```python
from build123d import *

# Parameters (mm, degrees)
SKETCH1_W               = 229
SKETCH1_H               = 15
BOSS_EXTRUDE1_DEPTH     = 3.375
M3_CLEARANCE_HOLE1_D    = 3.4
CUT_EXTRUDE1_DEPTH      = 116.527661731
CUT_EXTRUDE1_DEPTH_BACK = 116.527661731
SKETCH10_W              = 15
SKETCH10_H              = 1.6875


with BuildPart() as part:
    # Sketch1 → Boss-Extrude1 (new body)
    with BuildSketch(Plane(origin=(0, 0, 0), x_dir=(1, 0, 0), z_dir=(0, 1, 0))):
        Rectangle(SKETCH1_W, SKETCH1_H)
    extrude(amount=BOSS_EXTRUDE1_DEPTH)

    # M3 Clearance Hole1 (through all)
    with Locations(Plane(origin=(0, 0, 0), x_dir=(-1, 0, 0), z_dir=(0, -1, 0))):
        with Locations((57, 0), (-57, 0)):
            Hole(M3_CLEARANCE_HOLE1_D / 2)

    # Sketch10 → Cut-Extrude1 (cut, two sides: drawn at the far end of the back side and taken through both)
    with BuildSketch(Plane.XY.offset(7.5).offset(-CUT_EXTRUDE1_DEPTH_BACK)):
        with Locations((0, 2.53125)):
            Rectangle(SKETCH10_W, SKETCH10_H)
    extrude(amount=CUT_EXTRUDE1_DEPTH + CUT_EXTRUDE1_DEPTH_BACK, mode=Mode.SUBTRACT)


solid = part.part
```
Geometry: final body of the model. Coordinates: model frame, mm. Coordinates: 2 decimals unless noted, no trailing zeros. Order: outer loops, then holes, each group sorted by start corner. A loop starts at its lowest first (then second) coordinate and runs counter-clockwise, first axis right, second up. Notation, with made-up numbers: (73.25, 28.5) - (125.25, 28.5) arc R31 cw to (125.25, 52.5) - close; hole circle Ø10 at (24.5, 13). An arc over 180 degrees is marked (long way). Write each question's results on one line, items separated by ' | '.
1) Section A-A, the plane z = 3.75. Return loops of the section in (x, y) (1 decimal), plus the area to 3 significant figures.
Results list:
outline: (-114.5, 0) - (114.5, 0) - (114.5, 3.4) - (7.5, 3.4) - (7.5, 1.7) - (-7.5, 1.7) - (-7.5, 3.4) - (-114.5, 3.4) - close | area: 748 mm^2
2) Line query: line 1 (X direction, y = 0.8, z = -0.25); line 2 (Z direction, x = 57, y = 1.7); line 3 (X direction, y = 2.25, z = -5). Output: solid intervals per line, ascending. Write a range as from..to.
Results list:
line 1: -114.5..-58.68, -55.32..55.32, 58.68..114.5 | line 2: -7.5..-1.7, 1.7..7.5 | line 3: -114.5..-7.5, 7.5..114.5
3) Pull-direction query (X, two-part tool) for faces 1 (the flat face through (-62, 3.375, 0)), 2 (the flat face through (0, 1.688, 0)); classes: pulls with the +X half, pulls with the -X half, needs draft (parallel to the pull), parting line crosses it, or undercut.
Results list:
face 1: needs draft | face 2: undercut
